Can you work these out from the model? Positions are in its coordinate system, mm. Face numbers are marked on the shaded views. A direction names the side the tool comes from. Give positions to 0.01 mm unless a question says otherwise; leave off trailing zeros. Write each loop counter-clockwise with the first axis right and the second up, starting at its lowest first coordinate (ties: lowest second). Pieces come first, ordered by that corner, then holes.
1. If I drill on probe 1 along Z at (x, y) = (0, 35); probe 2 along X at (y, z) = (26.5, 0); probe 3 along X at (y, z) = (24, 0), over which ranges is the centre line in solid material (lowest first)?
2. I'm going to push flat-ended pins straight in: pin 1 (5 mm diameter, centred on x = 0, z = 0, fed in from -Y); pin 2 (2 mm diameter, centred on x = 28.5, y = 11, fed in from -Z); pin 3 (5 mm diameter, centred on y = 22.5, z = -13.5, fed in from +X); pin 4 (4 mm diameter, centred on y = 21.5, z = -1.5, fed in from +X). Where does each tip first touch, or does it pass through?
3. Thinking about a two-plate mould opening in X: for the marked faces 1, 2 and 3, which applies, pulls with the +X half, pulls with the -X half, needs draft (parallel to the pull), parting line crosses it, or undercut?
4. Suppose I cut it at C-C (y = 10). Please give me the cut outline in (x, z).
5. On a 3-axis mill with a long thin cutter (end or side, diameter ignored), from which of +Z, -Z, +X, -X, +Y, -Y can I reach the whole of each face in a straight line? I mean the marked faces 4, 5 and 6. Say none if no direction works.
Autodesk Inventor part; units mm, degrees
ref_plane "YZ Plane" through (0, 0, 0) normal (1, 0, 0) x (0, 1, 0)
ref_plane "XZ Plane" through (0, 0, 0) normal (0, 1, 0) x (-1, 0, 0)
ref_plane "XY Plane" through (0, 0, 0) normal (0, 0, 1) x (1, 0, 0)
sketch "Skizze5" plane through (0, 0, 0) normal (0, 0, 1) x (1, 0, 0)
  line L0 (0, 0) -> (14.5, 0)
  line L1 (33.3, 6) -> (50.9, 6)
  line L2 (33.3, 6) -> (23, 5.6403)
  arc A0 (23, 5.6403) -> (14.5, 0) centre (23.34, -4.0971) ccw
  line L3 (50.9, 6) -> (50.9, 7.3)
  line L4 (50.9, 7.3) -> (50.88, 7.3)
  line L5 (50.88, 7.3) -> (50.88, 13.3)
  line L6 (0, 0) -> (9.7, 0)
  line L7 (9.7, 0) -> (9.7, 48)
  line L8 (9.7, 48) -> (0, 48)
  line L9 (0, 48) -> (0, 0)
  line L10 (9.7, 48) -> (9.7, 41)
  line L11 (9.7, 41) -> (35.5, 41)
  line L12 (35.5, 41) -> (35.5, 17.4211)
  line L13 (50.88, 13.3) -> (35.5, 17.4211)
  arc A1 (35.5, 28.1636) -> (45.8765, 14.6407) centre (49.5, 28.1636) ccw
  line L14 (50.88, 13.3) -> (35.0608, 13.3)
  dimension "d21" = 14.5
  dimension "d22" = 50.9
  dimension "d23" = 6
  dimension "d24" = 33.3
  dimension "d25" = 23
  dimension "d26" = 2
  dimension "d28" = 1.3
  dimension "d29" = 0.02
  dimension "d30" = 6
  dimension "d31" = 9.7
  dimension "d32" = 48
  dimension "d33" = 7
  dimension "d47" = 25.8
  dimension "d48" = 35.5
  dimension "d49" = 105
  dimension "d53" = 14
  dimension "d54" = 15
  dimension "d55" = 35
revolve "Umdrehung1" add sketch "Skizze5" angle 360 about axis through (0, 48, 0) along (0, -1, 0)
sketch "Skizze6" plane through (0, 0, 0) normal (0, -1, 0) x (1, 0, 0)
  circle A0 centre (0, 0) radius 14.5
hole "Hole2" at (0, 0, 0) direction (0, 1, 0) diameter 8 end through all
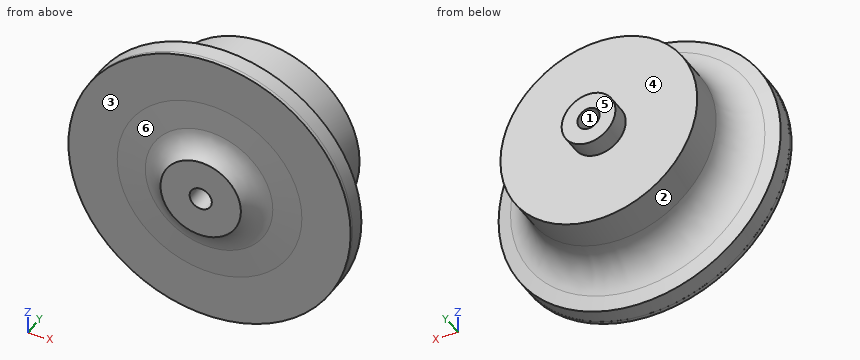
Checks:
1. probe 1: z = -35.5 to -4, 4 to 35.5
1. probe 2: x = -35.6 to -4, 4 to 35.6
1. probe 3: x = -36.13 to -4, 4 to 36.13
2. pin 1: passes through
2. pin 2: stops at z = -42.81
2. pin 3: stops at x = 35.86
2. pin 4: stops at x = 38.48
3. face 1: undercut
3. face 2: parting line crosses it
3. face 3: needs draft
4. outline: circle Ø101.76 at (0, 0); hole circle Ø8 at (0, 0)
5. face 4: +Y
5. face 5: +Z, -Z, +X, -X, +Y
5. face 6: -Y
